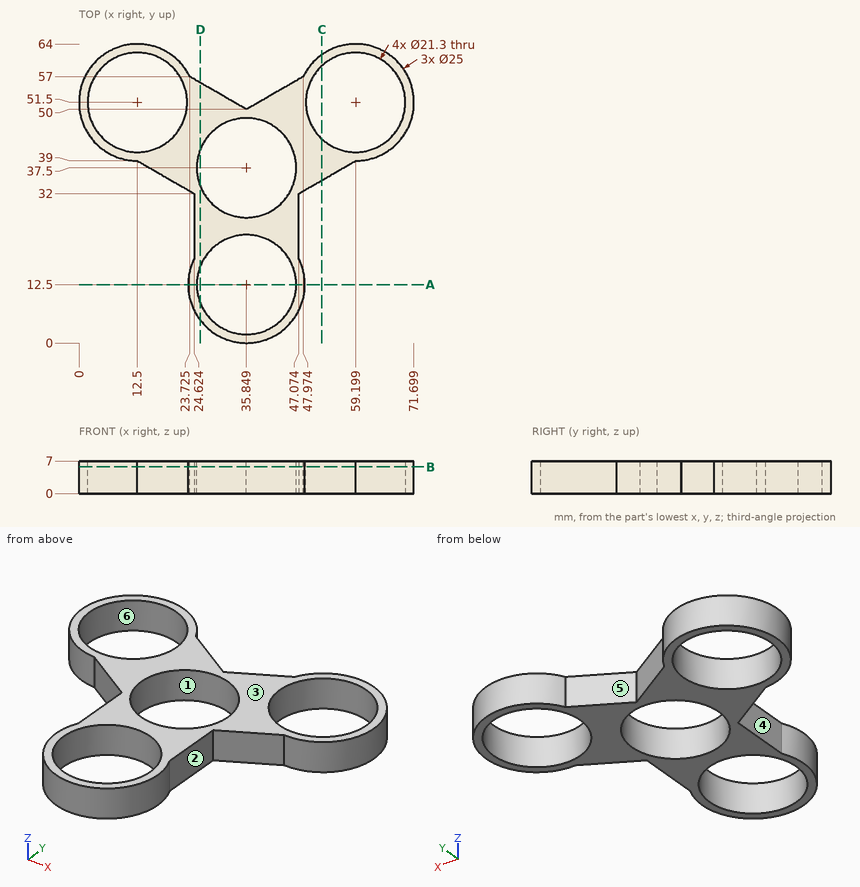
Answer from the drawing. Dimensions are ordinates in mm from the lowest x, y and z of the part. A direction names the side the tool comes from. Coordinates: 2 decimals unless noted, no trailing zeros. Write each loop counter-clockwise with the first axis right and the second up, starting at its lowest first coordinate (ties: lowest second). Pieces come first, ordered by that corner, then holes. Notation, with made-up numbers: (45, -16.5) - (91, -16.5) arc R7 ccw to (91, -12.5) - close; hole circle Ø5 at (-21, 49). An arc over 180 degrees is marked (long way). One line per question, with ' | ' between items.
Q1. Consider L1, parallel to X at y = 45, z = 6 (1 decimal); L2, parallel to X at y = 54.5, z = 2 (1 decimal); L3, parallel to Y at x = 32.5, z = 0.5 (1 decimal). Determine where each line is inside the solid, lowest interval first. Write a range as [from, to].
Result set:
L1: [1.8, 4.1], [20.9, 28.3], [43.4, 50.8], [67.6, 69.9] | L2: [0.4, 2.3], [22.7, 28.1], [43.6, 49], [69.4, 71.3] | L3: [0.5, 2.4], [22.6, 27.4], [47.6, 51.9]
Q2. Find section A-A, the plane y = 12.5. Write down the section's boundary in (x, z), plus the area to 3 significant figures.
Result set:
outline: (23.35, 0) - (25.2, 0) - (25.2, 7) - (23.35, 7) - close; (46.5, 0) - (48.35, 0) - (48.35, 7) - (46.5, 7) - close | area: 25.9 mm^2
Q3. Find section B-B, the plane z = 5.75. State how many separate pieces and enclosed holes the cut face has.
Result set:
separate pieces: 1 | enclosed holes: 4
Q4. For the marked faces 4, 5 and 6, determine the directions among +Z, -Z, +X, -X, +Y, -Y from which every point of the face is accessible in a straight line to the end or side of a thin tool.
Result set:
face 4: +Z, -Z, -X | face 5: +Z, -Z, +Y | face 6: +Z, -Z
Q5. Find section C-C, the plane x = 52. Write down the section's boundary in (y, z).
Result set:
outline: (34.84, 0) - (43.65, 0) - (43.65, 7) - (34.84, 7) - close; (59.35, 0) - (61.72, 0) - (61.72, 7) - (59.35, 7) - close
Q6. Each of these flat-tipped pins is pushed along its axis until it touches: P1, Ø3.5, axis at y = 26, z = 2.5, coming from the +X side; P2, Ø1, axis at x = 38, z = 5.5, coming from the +Y side; P3, Ø3.5, axis at y = 27.5, z = 4, coming from the -X side. Where does it stop, or does it pass through?
Result set:
P1: x = 47.07 | P2: y = 51.53 | P3: x = 24.62
Q7. Find section D-D, the plane x = 26. Write down the section's boundary in (y, z), plus the area to 3 significant figures.
Result set:
outline: (4.8, 0) - (8.45, 0) - (8.45, 7) - (4.8, 7) - close; (16.55, 0) - (33.45, 0) - (33.45, 7) - (16.55, 7) - close; (41.55, 0) - (55.69, 0) - (55.69, 7) - (41.55, 7) - close | area: 243 mm^2
Q8. Determine the mould class of the marked faces 1, 2 and 3 for opening direction X: +X half, -X half, draft (parallel to the pull), parting line (faces both ways), or undercut.
Result set:
face 1: undercut | face 2: +X half | face 3: draft
